from build123d import *

# Parameters (mm, degrees)
BOSS_EXTRUDE1_DEPTH     = 400
SKETCH2_W               = 100
SKETCH2_H               = 121
SKETCH2_W_2             = 95.3
SKETCH2_H_2             = 9.4
CUT_EXTRUDE1_DEPTH      = 268
CUT_EXTRUDE2_DEPTH      = 1
CUT_EXTRUDE2_DEPTH_BACK = 1311.69690242


with BuildPart() as part:
    # Sketch1 → Boss-Extrude1 (new body)
    with BuildSketch(Plane(origin=(0, 0, 0), x_dir=(0, 0, -1), z_dir=(1, 0, 0))):
        Polygon((0, 0), (-340, 0), (-350, 10), (-350, 960), (-310, 1000), (-203.251091608, 1000), (-203.251091608, 1310.69690242), (-108.48888922, 1310.69690242), (0, 1310.69690242), (0, 1000), (0, 970), (0, 820), (-9.396926208, 806.579798567), (-27.474774195, 800), (-190.603073792, 740.62615458), (-200, 727.205953147), (-200, 5), (0, 5), align=None)
    extrude(amount=BOSS_EXTRUDE1_DEPTH)

    # Sketch2 → Cut-Extrude1 (cut)
    with BuildSketch(Plane.XY.offset(350)):
        with Locations((200, 889.5)):
            Rectangle(SKETCH2_W, SKETCH2_H)
        with Locations((325, 889.5)):
            Rectangle(SKETCH2_W_2, SKETCH2_H_2)
    extrude(amount=-CUT_EXTRUDE1_DEPTH, mode=Mode.SUBTRACT)

    # Sketch3 → Cut-Extrude2 (cut, two sides)
    with BuildSketch(Plane(origin=(0, 0, 0), x_dir=(-1, 0, 0), z_dir=(0, -1, 0))) as cut_extrude2_sk:
        Polygon((32.971910004, -72.804395349), (-67.728153305, 29.569560354), (-322.648629759, 29.569560354), (-423.348693067, -72.804395349), (-423.348693067, 100.069531779), (32.971910004, 100.069531779), align=None)
    extrude(amount=CUT_EXTRUDE2_DEPTH, mode=Mode.SUBTRACT)
    extrude(cut_extrude2_sk.sketch, amount=-CUT_EXTRUDE2_DEPTH_BACK, mode=Mode.SUBTRACT)


solid = part.part
Could you check a few things on this model? Use its own coordinates, in mm. A direction names the side the tool comes from. Give positions to 0.01 mm unless a question says otherwise; leave off trailing zeros. Write each loop counter-clockwise with the first axis right and the second up, starting at its lowest first coordinate (ties: lowest second). Pieces come first, ordered by that corner, then holes. Notation, with made-up numbers: (63, -38) -> (83, -38) arc R32 cw to (83, -9) -> close; hole circle Ø7 at (-7.75, -35.75). An arc over 180 degrees is marked (long way). Write each question's results on one line, items separated by ' | '. Start each with the question number.
Q1. I'm going to push flat-ended pins straight in: pin 1 Ø6 at (x, y) = (305, 1062.5) entering from +Z; pin 2 Ø4.5 at (x, y) = (328, 889.5) entering from +Z; pin 3 Ø4 at (x, y) = (160.5, 404.5) entering from -Z. Where does each tip first touch, or does it pass through?
Q2. Suppose I cut it at B-B, the plane x = 222. List the corners of the cut face in (y, z) for me.
Q3. Suppose I cut it at C-C, the plane y = 1162.5. List the corners of the cut face in (x, z) for me.
Q4. Suppose I cut it at D-D, the plane z = 277.5. List the corners of the cut face in (x, y) for me, and give its area (3 significant figures).
Q5. Suppose I cut it at A-A, the plane z = 175.5. List the corners of the cut face in (x, y) for me, and give its area (3 significant figures).
Q6. Which directions (+Z, -Z, +X, -X, +Y, -Y) give clear straight access to the entire face, cutting with the end or side of a thin tool? Please do faces 1 (the face through (197, 371, 200)), 2 (the face through (250, 889, 218)), 3 (the face through (197, 1000, 257)).
Q7. I need wall thicknesses on probe 1 along Y at (x, z) = (179.5, 227); probe 2 along Y at (x, z) = (166.5, 126); probe 3 along Y at (x, z) = (302, 212). Which ranges of each line are inside material? Lowest first, please.
Q8. We'd pull the mould along X, two halves only. Please class faces 4 (the face through (199, 829, 218)), 5 (the face through (199, 950, 218)), 6 (the face through (193, 1062, 0)), 7 (the face through (375.53, 1047.79, 24.19)): +X half, -X half, draft (parallel to the pull), parting line (faces both ways), or undercut.
Outcome:
1) pin 1: z = 203.25 | pin 2: z = 82 | pin 3: z = 200
2) outline: (0, 0) -> (5, 0) -> (5, 200) -> (727.21, 200) -> (740.63, 190.6) -> (806.58, 9.4) -> (820, 0) -> (1310.7, 0) -> (1310.7, 203.25) -> (1000, 203.25) -> (1000, 310) -> (960, 350) -> (950, 350) -> (950, 82) -> (829, 82) -> (829, 350) -> (10, 350) -> (0, 340) -> close
3) outline: (0, 39.28) -> (38.64, 0) -> (351.73, 0) -> (400, 49.07) -> (400, 203.25) -> (0, 203.25) -> close
4) outline: (0, 0) -> (400, 0) -> (400, 1000) -> (0, 1000) -> close; hole (150, 829) -> (250, 829) -> (250, 950) -> (150, 950) -> close; hole (277.35, 884.8) -> (372.65, 884.8) -> (372.65, 894.2) -> (277.35, 894.2) -> close | area: 387,000 mm2
5) outline: (0, 0) -> (400, 0) -> (400, 5) -> (0, 5) -> close; (0, 746.12) -> (400, 746.12) -> (400, 1310.7) -> (0, 1310.7) -> close; hole (150, 829) -> (250, 829) -> (250, 950) -> (150, 950) -> close; hole (277.35, 884.8) -> (372.65, 884.8) -> (372.65, 894.2) -> (277.35, 894.2) -> close | area: 215,000 mm2
6) face 1: -Z, +X, -X | face 2: +Z | face 3: +Z, +X, -X, +Y
7) probe 1: 0 to 829, 950 to 1000 | probe 2: 0 to 5, 764.14 to 829, 950 to 1310.7 | probe 3: 0 to 884.8, 894.2 to 1000
8) face 4: undercut | face 5: undercut | face 6: draft | face 7: +X half
